Can you work these out from the drawing? Everything is in mm from the part's minimum corner. Give positions to 0.01 mm unless a question says otherwise; leave off trailing zeros. Write each loop counter-clockwise with the first axis right and the second up, starting at its lowest first coordinate (ties: lowest second). Pieces come first, ordered by that corner, then holes. Notation, with made-up numbers: (4, 41) - (54, 41) arc R23 ccw to (54, 53) - close; hole circle Ø8 at (64.5, 58.5). An arc over 180 degrees is marked (long way). Answer in a Markdown table with one row per item.
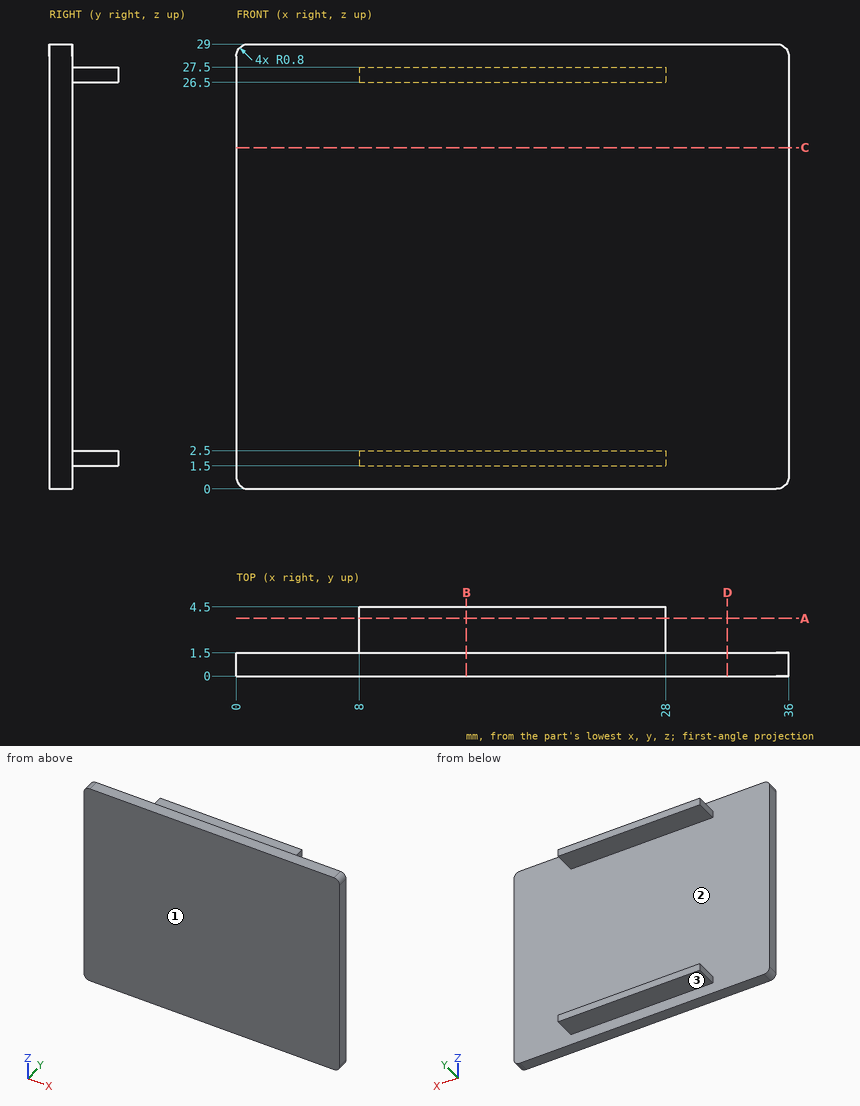
1) If I drill on line 1 (Z direction, x = 10.5, y = 4.2); line 2 (Y direction, x = 11, z = 19.5), over which ranges is the centre line in solid material (lowest first)?
Check values:
| item | result |
|---|---|
| line 1 | z = 1.5 to 2.5, 26.5 to 27.5 |
| line 2 | y = 0 to 1.5 |
2) Imagine slicing it at A-A (y = 3.75). List the corners of the cut face in (x, z) for me.
Check values:
| item | result |
|---|---|
| outline | (8, 1.5) - (28, 1.5) - (28, 2.5) - (8, 2.5) - close; (8, 26.5) - (28, 26.5) - (28, 27.5) - (8, 27.5) - close |
3) Will these pins go through, and if not, where does the flat tip stop? P1, Ø2.5, axis at x = 14, y = 3.5, coming from the +Z side; P2, Ø1.5, axis at x = 13.5, y = 3, coming from the -Z side; P3, Ø0.5, axis at y = 3.5, z = 27, coming from the -X side.
Check values:
| item | result |
|---|---|
| P1 | stops at z = 27.5 |
| P2 | stops at z = 1.5 |
| P3 | stops at x = 8 |
4) Imagine slicing it at D-D (x = 32). List the corners of the cut face in (y, z) for me, then the cut area to 3 significant figures.
Check values:
| item | result |
|---|---|
| outline | (0, 0) - (1.5, 0) - (1.5, 29) - (0, 29) - close |
| area | 43.5 mm2 |
5) Imagine slicing it at B-B (x = 15). List the corners of the cut face in (y, z) for me, then the cut area to 3 significant figures.
Check values:
| item | result |
|---|---|
| outline | (0, 0) - (1.5, 0) - (1.5, 1.5) - (4.5, 1.5) - (4.5, 2.5) - (1.5, 2.5) - (1.5, 26.5) - (4.5, 26.5) - (4.5, 27.5) - (1.5, 27.5) - (1.5, 29) - (0, 29) - close |
| area | 49.5 mm2 |
6) Imagine slicing it at C-C (z = 22.25). List the corners of the cut face in (x, y) for me.
Check values:
| item | result |
|---|---|
| outline | (0, 0) - (36, 0) - (36, 1.5) - (0, 1.5) - close |
7) We'd pull the mould along Z, two halves only. Please class the marked faces 1, 2 and 3: +Z half, -Z half, draft (parallel to the pull), parting line (faces both ways), or undercut.
Check values:
| item | result |
|---|---|
| face 1 | draft |
| face 2 | undercut |
| face 3 | -Z half |
